Geometry check sheet. Reference: the model listing, model coordinates, mm. A direction names the side the tool comes from. Coordinates: 2 decimals unless noted, no trailing zeros. Write each loop counter-clockwise with the first axis right and the second up, starting at its lowest first coordinate (ties: lowest second). Pieces come first, ordered by that corner, then holes.
from build123d import *

# Parameters (mm, degrees)
SKETCH_1_W      = 82.5
SKETCH_1_H      = 13
SKETCH_2_R      = 70
EXTRUDE_1_DEPTH = 5
SKETCH_3_R      = 50
EXTRUDE_2_DEPTH = 2.5
HOLE_WIZARD_2_D = 70
CHAMFER_1_SIZE  = 0.5


with BuildPart() as part:
    # 草圖1 → 旋轉1 (revolve)
    with BuildSketch(Plane(origin=(0, 0, 0), x_dir=(-1, 0, 0), z_dir=(0, 0, -1)), mode=Mode.PRIVATE) as revolve_1_sk:
        with Locations((-41.25, 13.5)):
            Rectangle(SKETCH_1_W, SKETCH_1_H)
    revolve(revolve_1_sk.sketch.rotate(Axis((0, 7, 0), (0, 1, 0)), 270), axis=Axis((0, 7, 0), (0, 1, 0)))

    # 草圖2 → 填料-伸長1 (add)
    with BuildSketch(Plane.XZ.offset(-7)):
        with Locations(Location((0, 0, 0), (0, 0, 270))):
            Circle(SKETCH_2_R)
    extrude(amount=EXTRUDE_1_DEPTH)

    # 草圖3 → 填料-伸長2 (add)
    with BuildSketch(Plane(origin=(0, 20, 0), x_dir=(-1, 0, 0), z_dir=(0, 1, 0))):
        with Locations(Location((0, 0, 0), (0, 0, 90))):
            Circle(SKETCH_3_R)
    extrude(amount=EXTRUDE_2_DEPTH)

    # 鑽孔2 (through all)
    with Locations(Plane(origin=(0, 22.5, 0), x_dir=(1, 0, 0), z_dir=(0, 1, 0))):
        with Locations((0, 0)):
            Hole(HOLE_WIZARD_2_D / 2)

    # 導角1
    chamfer_1_edges = [part.edges().sort_by_distance(p)[0] for p in [
        (0, 2, 70),
        (0, 22.5, -50),
        (35, 22.5, 0),
        (35, 2, 0),
        (0, 20, -82.5),
        (0, 7, -82.5),
    ]]
    chamfer(chamfer_1_edges, length=CHAMFER_1_SIZE)


solid = part.part
1. Gauge pin test, flat ends, axial feed: pin 1 Ø1.5 at (y, z) = (5, 61.5) entering from +X; pin 2 Ø5 at (y, z) = (11.5, -19) entering from -X; pin 3 Ø10 at (y, z) = (11.5, -46.5) entering from -X. Record the tip position at first contact, or that the pin passes through.
Computed values:
pin 1: stops at x = 34.78
pin 2: stops at x = -80.83
pin 3: stops at x = -71.3
2. Sectioned sample at C-C, the plane y = 11.5. Record the boundary of the cut face in (x, z), and give its area (3 significant figures).
Computed values:
outline: circle Ø165 at (0, 0); hole circle Ø70 at (0, 0)
area: 17,500 mm2
3. Access from +Z, -Z, +X, -X, +Y, -Y to the whole of each face (thin tool, end or side, straight path). Record for faces 4 (the cylindrical face through (-80.54, 13.58, -17.88)), 5 (the cylindrical face through (15.02, 20.99, 47.69)), 6 (the flat face through (37, 7, 60)).
Computed values:
face 4: +Y, -Y
face 5: +Y
face 6: -Y
4. Thickness scan on line 1 along X through (y, z) = (14.5, 0); line 2 along Y through (x, z) = (-64, -2.5); line 3 along Z through (x, y) = (-26.5, 18.5). Record the ranges inside material, lowest first.
Computed values:
line 1: x = -82.5 to -35, 35 to 82.5
line 2: y = 2 to 20
line 3: z = -78.13 to -22.86, 22.86 to 78.13
5. Sectioned sample at B-B, the plane z = 0. Record the boundary of the cut face in (x, y), and give its area (3 significant figures).
Computed values:
outline: (-82.5, 7.5) - (-82, 7) - (-70, 7) - (-70, 2.5) - (-69.5, 2) - (-35.5, 2) - (-35, 2.5) - (-35, 22) - (-35.5, 22.5) - (-49.5, 22.5) - (-50, 22) - (-50, 20) - (-82, 20) - (-82.5, 19.5) - close; (35, 2.5) - (35.5, 2) - (69.5, 2) - (70, 2.5) - (70, 7) - (82, 7) - (82.5, 7.5) - (82.5, 19.5) - (82, 20) - (50, 20) - (50, 22) - (49.5, 22.5) - (35.5, 22.5) - (35, 22) - close
area: 1,660 mm2
6. Sectioned sample at A-A, the plane x = 0. Record the boundary of the cut face in (y, z), and give its area (3 significant figures).
Computed values:
outline: (2, -69.5) - (2.5, -70) - (7, -70) - (7, -82) - (7.5, -82.5) - (19.5, -82.5) - (20, -82) - (20, -50) - (22, -50) - (22.5, -49.5) - (22.5, -35.5) - (22, -35) - (2.5, -35) - (2, -35.5) - close; (2, 35.5) - (2.5, 35) - (22, 35) - (22.5, 35.5) - (22.5, 49.5) - (22, 50) - (20, 50) - (20, 82) - (19.5, 82.5) - (7.5, 82.5) - (7, 82) - (7, 70) - (2.5, 70) - (2, 69.5) - close
area: 1,660 mm2
7. Draft check along Z on faces 1 (the cylindrical face through (-42.594, 4.781, 55.55)), 2 (the flat face through (34, 22.5, -12)), 3 (the cylindrical face through (28, 12, 21)). Enter one of: released by +Z, released by -Z, zero draft, split by the parting line, or undercut.
Computed values:
face 1: split by the parting line
face 2: zero draft
face 3: undercut
